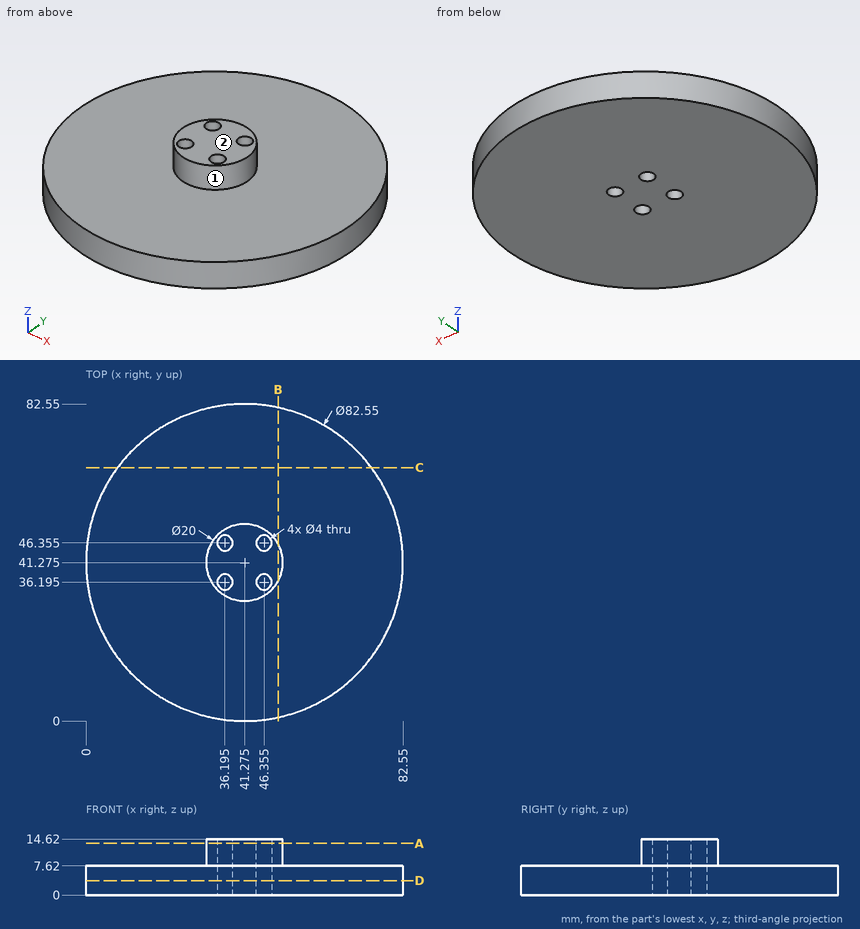
Can you work these out from the drawing? Everything is in mm from the part's minimum corner. A direction names the side the tool comes from. Round coordinates to 2 decimals unless told otherwise and drop trailing zeros. Loops run counter-clockwise (first coordinate to the right, second up) from the corner with the lowest first, then second, coordinate; pieces in that order, holes last. Notation, with made-up numbers: (78, -25.5) -> (86, -25.5) arc R5 cw to (86, -18.5) -> close; hole circle Ø5 at (62, 6). An arc over 180 degrees is marked (long way). Answer in a Markdown table with one row per item.
Item 1: Suppose I cut it at A-A, the plane z = 13.5. List the corners of the cut face in (x, y) for me (1 decimal), plus the area to 3 significant figures.
Answer block:
| item | result |
|---|---|
| outline | circle Ø20 at (41.3, 41.3); hole circle Ø4 at (36.2, 36.2); hole circle Ø4 at (36.2, 46.4); hole circle Ø4 at (46.4, 36.2); hole circle Ø4 at (46.4, 46.4) |
| area | 264 mm² |
Item 2: If I drill on probe 1 along X at (y, z) = (47, 3.5); probe 2 along Z at (x, y) = (20.5, 50.5); probe 3 along Y at (x, z) = (7, 6.25), over which ranges is the centre line in solid material (lowest first)?
Answer block:
| item | result |
|---|---|
| probe 1 | 0.4 to 34.3, 38.09 to 44.46, 48.25 to 82.15 |
| probe 2 | 0 to 7.62 |
| probe 3 | 18.28 to 64.27 |
Item 3: Will these pins go through, and if not, where does the flat tip stop? P1, Ø1.5, axis at x = 18, y = 57.5, coming from the +Z side; P2, Ø1.5, axis at x = 71, z = 7, coming from the +Y side; P3, Ø1.5, axis at x = 16, z = 4.5, coming from the +Y side.
Answer block:
| item | result |
|---|---|
| P1 | z = 7.62 |
| P2 | y = 70.67 |
| P3 | y = 74.47 |
Item 4: Suppose I cut it at C-C, the plane y = 66. List the corners of the cut face in (x, z) for me (1 decimal), plus the area to 3 significant figures.
Answer block:
| item | result |
|---|---|
| outline | (8.2, 0) -> (74.3, 0) -> (74.3, 7.6) -> (8.2, 7.6) -> close |
| area | 504 mm² |
Item 5: Suppose I cut it at B-B, the plane x = 50. List the corners of the cut face in (y, z) for me, plus the area to 3 significant figures.
Answer block:
| item | result |
|---|---|
| outline | (0.93, 0) -> (81.62, 0) -> (81.62, 7.62) -> (46.16, 7.62) -> (46.16, 14.62) -> (36.39, 14.62) -> (36.39, 7.62) -> (0.93, 7.62) -> close |
| area | 683 mm² |
Item 6: Suppose I cut it at D-D, the plane z = 3.75. Give the number of separate pieces and of enclosed holes in the cut face, plus the area to 3 significant figures.
Answer block:
| item | result |
|---|---|
| separate pieces | 1 |
| enclosed holes | 4 |
| area | 5,300 mm² |
Item 7: On a 3-axis mill with a long thin cutter (end or side, diameter ignored), from which of +Z, -Z, +X, -X, +Y, -Y can I reach the whole of each face in a straight line? I mean the marked faces 1 and 2. Say none if no direction works.
Answer block:
| item | result |
|---|---|
| face 1 | +Z |
| face 2 | +Z, +X, -X, +Y, -Y |
